Here's how the part is built. I have some questions about the finished solid (model axes, mm). Face numbers are marked on the shaded views. Give positions to 0.01 mm unless a question says otherwise; leave off trailing zeros. Write each loop counter-clockwise with the first axis right and the second up, starting at its lowest first coordinate (ties: lowest second). Pieces come first, ordered by that corner, then holes. Notation, with made-up numbers: (-26.5, 10.5) - (-19.5, 10.5) arc R13 cw to (-19.5, 35.5) - close; hole circle Ø4 at (55.25, -31). An arc over 180 degrees is marked (long way). One line per item, written item: value. Start each with the question number.
1) Please list where these lines run through material, in increasing order: L1, parallel to Y at x = 4, z = 4.75; L2, parallel to Z at x = -9, y = 2; L3, parallel to X at y = 3.05, z = 0. Write a range as [from, to].
2) I'm going to push flat-ended pins straight in: P1, Ø1, axis at x = -6, z = -4.5, coming from the +Y side; P2, Ø8.5, axis at x = 0, z = 0, coming from the -Y side. Where does each tip first touch, or does it pass through?
3) Imagine slicing it at C-C on y = 2.2. Write out the boundary of the cut face in (x, z).
4) We'd pull the mould along X, two halves only. Please class the marked faces 1 and 2: +X half, -X half, draft (parallel to the pull), parting line (faces both ways), or undercut.
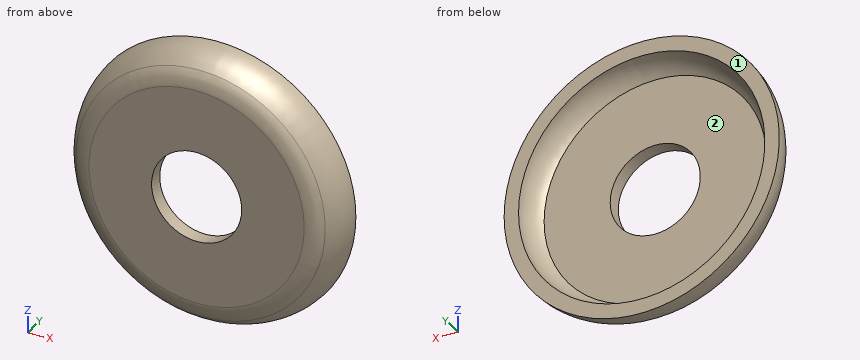
from build123d import *


with BuildPart() as part:
    # Sketch2 → Revolve1 (revolve)
    with BuildSketch(Plane.XY):
        with BuildLine():
            Line((4.7625, 0), (11.371782512, 0))
            ThreePointArc((11.371782512, 0), (12.345828047, 0.194187711), (13.170938407, 0.747058824))
            ThreePointArc((13.170938407, 0.747058824), (14.185363864, 2.26952669), (14.5415, 4.064))
            Line((14.5415, 4.064), (13.0175, 4.064))
            ThreePointArc((13.0175, 4.064), (12.682306331, 2.644096834), (11.7475, 1.524))
            Line((11.7475, 1.524), (4.7625, 1.524))
            Line((4.7625, 1.524), (4.7625, 0))
        make_face()
    revolve(axis=Axis((0, 0, 0), (0, 1, 0)))


solid = part.part
Numbers:
1. L1: [0, 1.52]
1. L2: [-10.81, -8.32], [8.32, 10.81]
1. L3: [-14.43, -12.85], [12.85, 14.43]
2. P1: y = 1.52
2. P2: through
3. outline: circle Ø28.31 at (0, 0); hole circle Ø24.83 at (0, 0)
4. face 1: draft
4. face 2: undercut
